Here's how the part is built. I have some questions about the finished solid (model axes, mm). A direction names the side the tool comes from. Round coordinates to 2 decimals unless told otherwise and drop trailing zeros. Write each loop counter-clockwise with the first axis right and the second up, starting at its lowest first coordinate (ties: lowest second). Pieces come first, ordered by that corner, then holes. Notation, with made-up numbers: (48, -11.75) -> (87, -11.75) arc R15 ccw to (87, 3.25) -> close; hole circle Ø4 at (0.5, -11.75). An arc over 180 degrees is marked (long way). Put each result on its own line as item: value. Start each with the question number.
1. Suppose I cut it at B-B (x = 65). Please give me the cut outline in (y, z).
2. Suppose I cut it at D-D (x = 76). Please give me the cut outline in (y, z).
3. We'd pull the mould along Y, two halves only. Please class faces 1 (the face through (69.283, 30.07, -0.833)), 2 (the face through (60.73, 40.88, 11.62)), 3 (the face through (19.56, 55.24, -43.07)), 4 (the face through (68.14, 21.01, -33.59)): +Y half, -Y half, draft (parallel to the pull), parting line (faces both ways), or undercut.
4. Suppose I cut it at C-C (z = -19). Please give me the cut outline in (x, y).
5. Which directions (+Z, -Z, +X, -X, +Y, -Y) give clear straight access to the entire face, cutting with the end or side of a thin tool? Please do faces 5 (the face through (60.725, 38.054, -6.143)), 6 (the face through (0, 62, -44)), 7 (the face through (52.295, 21.014, -32.372)).
6. For pin 1 (8.5 mm diameter, centred on x = 47.75, z = -33.8, fed in from -Y); pin 2 (1 mm diameter, centred on x = 70, z = -1, fed in from +Y); pin 3 (11 mm diameter, centred on x = 65, y = 46, fed in from +Z), each with a flat end and sliding along its axis, tell me the tip position at first contact or that it passes through.
7. I need wall thicknesses on probe 1 along Z at (x, y) = (70, 25.5); probe 2 along Y at (x, z) = (48, -52); probe 3 along X at (y, z) = (40.5, -57). Which ranges of each line are inside material? Lowest first, please. Write a range as from..to.
8. Suppose I cut it at A-A (x = 35). Please give me the cut outline in (y, z).
```python
from build123d import *

# Parameters (mm, degrees)
BOSS_EXTRUDE1_DEPTH   = 44.45
SKETCH3_R             = 9.525
CUT_EXTRUDE1_DEPTH    = 6.35
BOSS_EXTRUDE2_DEPTH   = 57.15
SKETCH5_R             = 9.525
CUT_EXTRUDE2_DEPTH    = 6.35
SKETCH6_R             = 4.7625
CUT_EXTRUDE3_DEPTH    = 12.7
BODY_MOVE_COPY1_ANGLE = 180


with BuildPart() as part:
    # Sketch1 → Boss-Extrude1 (new body)
    with BuildSketch(Plane(origin=(0, 0, 0), x_dir=(1, 0, 0), z_dir=(0, 1, 0))):
        Polygon((57.15, 0), (88.9, 0), (88.9, 6.35), (57.15, 24.680871047), (57.15, 50.8), (0, 50.8), (0, 0), align=None)
    extrude(amount=BOSS_EXTRUDE1_DEPTH)

    # Sketch3 → Cut-Extrude1 (cut)
    with BuildSketch(Plane(origin=(24.974630657, 0, -43.257329198), x_dir=(-0.866025404, 0, -0.5), z_dir=(0.5, 0, -0.866025404))):
        with Locations((-54.764658396, 22.352)):
            Circle(SKETCH3_R)
    extrude(amount=-CUT_EXTRUDE1_DEPTH, mode=Mode.SUBTRACT)

    # Sketch4 → Boss-Extrude2 (add)
    with BuildSketch(Plane.ZY):
        Polygon((-50.8, 44.45), (-30.099, 80.305183767), (-19.100477372, 73.955183767), (-36.135303163, 44.45), (0, 44.45), (0, 0), (-50.8, 0), align=None)
    extrude(amount=-BOSS_EXTRUDE2_DEPTH)

    # Sketch5 → Cut-Extrude2 (cut)
    with BuildSketch(Plane(origin=(0, 33.109545256, -57.347414599), x_dir=(-1, 0, 0), z_dir=(0, 0.5, -0.866025404))):
        with Locations((-28.702, 35.446829198)):
            Circle(SKETCH5_R)
    extrude(amount=-CUT_EXTRUDE2_DEPTH, mode=Mode.SUBTRACT)

    # Sketch6 → Cut-Extrude3 (cut)
    with BuildSketch(Plane(origin=(0, 0, -50.8), x_dir=(-1, 0, 0), z_dir=(0, 0, -1))):
        with Locations((-41.148, 31.75)):
            Circle(SKETCH6_R)
        with Locations((-16.002, 31.75)):
            Circle(SKETCH6_R)
        with Locations((-16.002, 12.7)):
            Circle(SKETCH6_R)
        with Locations((-41.148, 12.7)):
            Circle(SKETCH6_R)
    extrude(amount=-CUT_EXTRUDE3_DEPTH, mode=Mode.SUBTRACT)


with BuildPart() as part_1:
    # Body-Move/Copy1: moved
    add(part.part.moved(Location((0, 0, 0))).rotate(Axis((44.45, 32.776295942, -32.776295942), (0, 0.707106781, 0.707106781)), BODY_MOVE_COPY1_ANGLE))


solid = part_1.part
```
Verdict:
1. outline: (14.75, -65.55) -> (65.55, -65.55) -> (65.55, -21.1) -> (29.42, -21.1) -> (46.45, 8.4) -> (35.45, 14.75) -> (30.04, 5.38) -> (35.54, 2.2) -> (27.31, -12.04) -> (21.82, -8.87) -> (14.75, -21.1) -> close
2. outline: (14.75, -65.55) -> (65.55, -65.55) -> (65.55, -21.1) -> (29.42, -21.1) -> (46.45, 8.4) -> (35.45, 14.75) -> (14.75, -21.1) -> (14.75, -30.19) -> (27.45, -30.19) -> (27.45, -37.42) -> (14.75, -37.42) -> (14.75, -49.24) -> (27.45, -49.24) -> (27.45, -56.47) -> (14.75, -56.47) -> close
3. face 1: undercut
3. face 2: +Y half
3. face 3: undercut
3. face 4: draft
4. outline: (31.75, 15.97) -> (88.9, 15.97) -> (88.9, 30.63) -> (31.75, 30.63) -> close
5. face 5: +X, -X, +Y
5. face 6: +Z, -Z, -X, +Y, -Y
5. face 7: -Y
6. pin 1: stops at y = 27.45
6. pin 2: stops at y = 41.31
6. pin 3: stops at z = 11.84
7. probe 1: z = -65.55..-56.63, -49.07..-37.58, -30.02..-2.49
7. probe 2: y = 27.45..65.55
7. probe 3: x = 31.75..88.9
8. outline: (14.75, -65.55) -> (65.55, -65.55) -> (65.55, -21.1) -> (29.42, -21.1) -> (46.45, 8.4) -> (35.45, 14.75) -> (14.75, -21.1) -> close
